Here's how the part is built. I have some questions about the finished solid (model axes, mm). Coordinates: 2 decimals unless noted, no trailing zeros. Write each loop counter-clockwise with the first axis right and the second up, starting at its lowest first coordinate (ties: lowest second). Pieces come first, ordered by that corner, then holes.
from build123d import *


with BuildPart() as part:
    # Esquisse2 → Révolution1 (revolve)
    with BuildSketch(Plane(origin=(0, 0, 0), x_dir=(0, 0, -1), z_dir=(1, 0, 0)), mode=Mode.PRIVATE) as r_volution1_sk:
        Polygon((2, 1.5), (-2, 1.5), (-2, 2.5), (-1.574731183, 2.5), (-1.574731183, 2.75672043), (-1.9, 2.75672043), (-1.9, 3.25672043), (-1.510215054, 3.646505376), (-1.9, 3.646505376), (-1.9, 4), (-2, 4), (-2, 5), (2, 5), (2, 4), (1.9, 4), (1.9, 3.646505376), (1.510215054, 3.646505376), (1.9, 3.25672043), (1.9, 2.75672043), (1.574731183, 2.75672043), (1.574731183, 2.5), (2, 2.5), align=None)
    revolve(r_volution1_sk.sketch.rotate(Axis((0, 0, 4.422043011), (0, 0, -1)), 90), axis=Axis((0, 0, 4.422043011), (0, 0, -1)))


solid = part.part
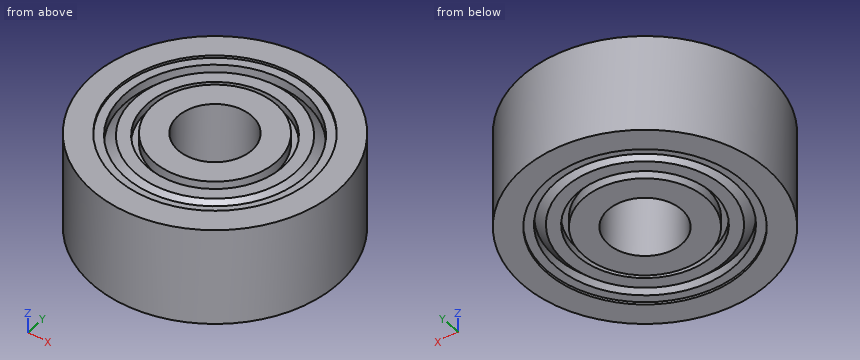
1. If I drill on line 1 (Y direction, x = 0, z = 1.95); line 2 (Y direction, x = 0, z = -1.7); line 3 (Y direction, x = 0, z = -1.85), over which ranges is the centre line in solid material (lowest first)?
2. For pin 1 Ø1 at (y, z) = (3, -1.5) entering from +X, with a flat end and sliding along its axis, tell me the tip position at first contact or that it passes through.
3. I want a section at A-A (z = -0.8). List the corners of the cut face in (x, y) for me, then the cut area to 3 significant figures.
Response values:
1. line 1: y = -5 to -4, -2.5 to -1.5, 1.5 to 2.5, 4 to 5
1. line 2: y = -5 to -3.65, -3.46 to -2.76, -2.5 to -1.5, 1.5 to 2.5, 2.76 to 3.46, 3.65 to 5
1. line 3: y = -5 to -3.65, -3.31 to -2.76, -2.5 to -1.5, 1.5 to 2.5, 2.76 to 3.31, 3.65 to 5
2. pin 1: stops at x = 4.33
3. outline: circle Ø10 at (0, 0); hole circle Ø3 at (0, 0)
3. area: 71.5 mm2
